Read the model definition and answer for the solid it produces. Units are mm, in the model's axes. Face numbers are marked on the shaded views. A direction names the side the tool comes from. Round coordinates to 2 decimals unless told otherwise and drop trailing zeros. Write each loop counter-clockwise with the first axis right and the second up, starting at its lowest first coordinate (ties: lowest second). Pieces come first, ordered by that corner, then holes.
from build123d import *

# Parameters (mm, degrees)
F0_W     = 30
F0_H     = 46
F1_DEPTH = 70
F2_W     = 22.8
F2_H     = 30
F3_DEPTH = 70
F4_R     = 2.2
F5_DEPTH = 3.6
F6_R     = 5


with BuildPart() as f1:
    # F0 (on Front) → F1 (new body)
    with BuildSketch(Plane.XZ):
        with Locations((7.198161, 6.185042)):
            Rectangle(F0_W, F0_H)
    extrude(amount=F1_DEPTH)

    # F2 (on face) → F3 (cut)
    with BuildSketch(Plane.XZ.offset(70)):
        with BuildLine():
            ThreePointArc((18.598161, 13.185042), (7.198161, 24.585042), (-4.201839, 13.185042))
            Line((-4.201839, 13.185042), (18.598161, 13.185042))
        make_face()
        with Locations((7.198161, -1.814958)):
            Rectangle(F2_W, F2_H)
    extrude(amount=-F3_DEPTH, mode=Mode.SUBTRACT)

    # F4 (on face) → F5 (cut, through all)
    with BuildSketch(Plane.YZ.offset(22.198161)):
        with Locations((-54.21123, 0)):
            Circle(F4_R)
        with Locations((-13.479018, 0)):
            Circle(F4_R)
    extrude(amount=-F5_DEPTH, mode=Mode.SUBTRACT)

    # F6
    f6_edges = [f1.edges().sort_by_distance(p)[0] for p in [
        (-7.801839, -35, 29.185042),
        (22.198161, -35, 29.185042),
    ]]
    fillet(f6_edges, radius=F6_R)


solid = f1.part
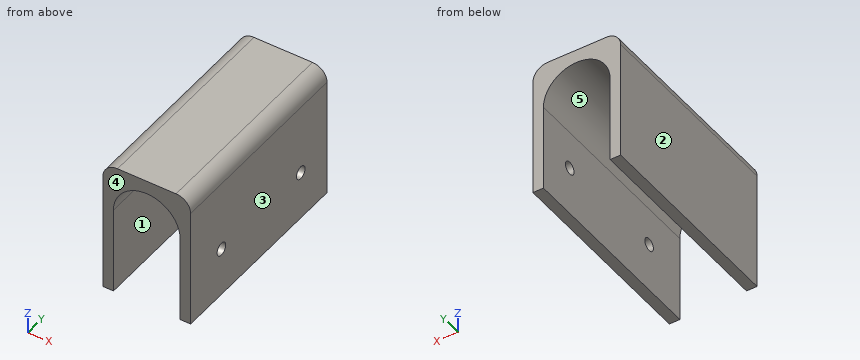
Q1. Which of the six approach directions +Z, -Z, +X, -X, +Y, -Y give full straight-line access (tool end or side, diameter ignored) to the marked faces 1 and 2?
Verdict:
face 1: -Z, +Y, -Y
face 2: +Z, -Z, -X, +Y, -Y
Q2. Straight lines are drawn through the part: probe 1 along X at (y, z) = (-59, 11.5); probe 2 along Z at (x, y) = (4.25, -52.5); probe 3 along X at (y, z) = (-15, 1). For each, find the intervals that lie inside material, in ascending order.
Verdict:
probe 1: x = -7.8 to -4.2, 18.6 to 22.2
probe 2: z = 24.2 to 29.19
probe 3: x = -7.8 to -4.2
Q3. Section D-D (x = 0.25) is taken. Determine the outline of the cut face in (y, z), then the cut area to 3 significant figures.
Verdict:
outline: (-70, 22.22) - (0, 22.22) - (0, 29.19) - (-70, 29.19) - close
area: 487 mm2
Q4. Flat-ended cylindrical pins translate along their axes: pin 1 Ø1 at (x, y) = (13.5, -35) entering from -Z; pin 2 Ø12 at (x, z) = (5, 7) entering from -Y; pin 3 Ø4 at (x, y) = (6, -42.5) entering from -Z. Find the tip coordinate at first contact, or state that the pin passes through.
Verdict:
pin 1: stops at z = 22.33
pin 2: passes through
pin 3: stops at z = 24.13
Q5. Determine the mould class of the marked faces 3, 4 and 5 for opening direction X: pulls with the +X half, pulls with the -X half, needs draft (parallel to the pull), parting line crosses it, or undercut.
Verdict:
face 3: pulls with the +X half
face 4: needs draft
face 5: undercut
Q6. Section B-B (z = 0) is taken. Determine the outline of the cut face in (x, y).
Verdict:
outline: (-7.8, -70) - (-4.2, -70) - (-4.2, 0) - (-7.8, 0) - close; (18.6, -70) - (22.2, -70) - (22.2, -56.41) - (18.6, -56.41) - close; (18.6, -52.01) - (22.2, -52.01) - (22.2, -15.68) - (18.6, -15.68) - close; (18.6, -11.28) - (22.2, -11.28) - (22.2, 0) - (18.6, 0) - close
Q7. Section A-A (z = 7.5) is taken. Determine the outline of the cut face in (x, y), then the cut area to 3 significant figures.
Verdict:
outline: (-7.8, -70) - (-4.2, -70) - (-4.2, 0) - (-7.8, 0) - close; (18.6, -70) - (22.2, -70) - (22.2, 0) - (18.6, 0) - close
area: 504 mm2
Q8. Section C-C (y = -10) is taken. Determine the outline of the cut face in (x, z).
Verdict:
outline: (-7.8, -16.81) - (-4.2, -16.81) - (-4.2, 13.19) arc R11.4 cw to (18.6, 13.19) - (18.6, -16.81) - (22.2, -16.81) - (22.2, 24.19) arc R5 ccw to (17.2, 29.19) - (-2.8, 29.19) arc R5 ccw to (-7.8, 24.19) - close
